Geometry: final body of the model. Coordinates: model frame, mm. Round coordinates to 2 decimals unless told otherwise and drop trailing zeros. Order: outer loops, then holes, each group sorted by start corner. A loop starts at its lowest first (then second) coordinate and runs counter-clockwise, first axis right, second up. Notation, with made-up numbers: M 56.5,-25 L 106.5,-25 A34 cw 106.5,5 Z; hole C 29,59.5 d9. An arc over 180 degrees is marked long. Put each result on its own line as item: value. Start each with the question number.
1) Section C-C, the plane z = -430.5. Return loops of the section in (x, y), then the cut area to 3 significant figures.
2) Section B-B, the plane y = -74.5. Return loops of the section in (x, z).
3) Material intervals for probe 1 along Z at (x, y) = (1.25, -49.5); probe 2 along Y at (x, z) = (0, -421); probe 3 along Z at (x, y) = (2.75, -54.5), sorted ascending. Write a range as [from, to].
4) First-contact query: P1, Ø2, axis at x = -2.5, y = -54.5, coming from the -Z side; P2, Ø1, axis at x = -1.5, z = -365.5, coming from the +Y side; P3, Ø5, axis at x = -3, y = -51, coming from the -Z side. Flat tips, straight axial feed; report the tip coordinate or a pass-through.
5) Section A-A, the plane x = -1. Return loops of the section in (y, z).
Autodesk Inventor part; units mm, degrees
ref_plane "YZ Plane" through (0, 0, 0) normal (1, 0, 0) x (0, 1, 0)
ref_plane "XZ Plane" through (0, 0, 0) normal (0, 1, 0) x (-1, 0, 0)
ref_plane "XY Plane" through (0, 0, 0) normal (0, 0, 1) x (1, 0, 0)
sketch "Sketch1" plane through (0, 0, 0) normal (0, 1, 0) x (-1, 0, 0)
  line L0 (0, 0) -> (0, -180) construction
  line L1 (5, 0) -> (5, -180)
  line L2 (-5, -180) -> (-5, 0)
  arc A0 (5, 0) -> (-5, 0) centre (0, 0) ccw
  arc A1 (-5, -180) -> (5, -180) centre (0, -180) ccw
  circle A2 centre (0, 0) radius 1.65
  line L3 (0, -40) -> (0, -140) construction
  line L4 (1.65, -40) -> (1.65, -140)
  line L5 (-1.65, -140) -> (-1.65, -40)
  arc A3 (1.65, -40) -> (-1.65, -40) centre (0, -40) ccw
  arc A4 (-1.65, -140) -> (1.65, -140) centre (0, -140) ccw
  point P0 (0, -90)
  point P1 (0, -90)
  dimension "d0" = 180
  dimension "d1" = 10
  dimension "d2" = 3.3
  dimension "d3" = 40
  dimension "d5" = 140
  dimension "d6" = 3.3
extrude "Extrusion1" add sketch "Sketch1" along normal blind 6
sketch "Sketch2" plane through (5, 0, 0) normal (1, 0, 0) x (0, 0, -1)
  line L0 (180, 0) -> (180, 6)
  line L1 (0, 0) -> (180, 0)
  line L2 (180, 0) -> (180, 6)
  line L3 (0, 6) -> (180, 6)
  line L4 (0, 0) -> (0, 6)
  line L5 (180, 0) -> (180, 0)
  line L6 (180, 0) -> (180, 6)
  line L7 (180, 6) -> (180, 6)
  line L8 (180, 0) -> (180, 6)
  line L9 (180, 0) -> (0, 0)
  arc A0 (498.004, -84) -> (180, 0) centre (180, -643.9437) ccw
  line L10 (180, 6) -> (0, 6)
  arc A1 (498.004, -78) -> (180, 6) centre (180, -637.9437) ccw
  line L11 (498.004, -78) -> (498.004, -84)
  line L12 (0, 0) -> (180, 0)
  dimension "d9" = 6
  dimension "d10" = 498.004
  dimension "d11" = 90
extrude "Extrusion2" add sketch "Sketch2" against normal blind 10 contours L0 A1 L11 A0
fillet "Fillet1" radius 2 4 edges at (0, -78, -498.004) (5, -81, -498.004) (-5, -81, -498.004) (0, -84, -498.004)
sketch "Sketch3" plane through (0, 6, 0) normal (0, 1, 0) x (1, 0, 0)
  line L0 (-25.1236, -17.4365) -> (19.1239, -17.4365)
  line L1 (19.1239, -17.4365) -> (19.1239, 173.8027)
  line L2 (19.1239, 173.8027) -> (-25.1236, 173.8027)
  line L3 (-25.1236, 173.8027) -> (-25.1236, -17.4365)
  line L4 (-48.0471, -35.7333) -> (42.457, -35.7333)
  line L5 (42.457, -35.7333) -> (42.457, 337.7497)
  line L6 (42.457, 337.7497) -> (-48.0471, 337.7497)
  line L7 (-48.0471, 337.7497) -> (-48.0471, -35.7333)
  line L8 (-102.0639, -92.3443) -> (98.6132, -92.3443)
  line L9 (98.6132, -92.3443) -> (98.6132, 617.9416)
  line L10 (98.6132, 617.9416) -> (-102.0639, 617.9416)
  line L11 (-102.0639, 617.9416) -> (-102.0639, -92.3443)
  point P0 (0, 0)
extrude "Extrusion3" cut sketch "Sketch3" against normal blind 100 contours L3 L2 L1 L0 | L7 L6 L5 L4
properties part number "Part_8_p1"
Result sheet:
1. outline: M -5,-50.72 L 5,-50.72 L 5,-44.72 L -5,-44.72 Z
1. area: 60.0 mm2
2. outline: M -5,-491.76 L 5,-491.76 L 5,-480.66 L -5,-480.66 Z
3. probe 1: z = [-441.53, -427.59]
3. probe 2: y = [-46.8, -40.8]
3. probe 3: z = [-452.5, -439.27]
4. P1: stops at z = -454.63
4. P2: stops at y = -21.15
4. P3: stops at z = -450.35
5. outline: M -82.32,-495.03 A2 ccw -80.57,-498 L -79.17,-498 A2 ccw -77.42,-496.99 A643.94 ccw -13.62,-337.75 L -19.62,-337.75 A643.94 cw Z
